Autodesk Inventor part; units mm, degrees
ref_plane "YZ Plane" through (0, 0, 0) normal (1, 0, 0) x (0, 1, 0)
ref_plane "XZ Plane" through (0, 0, 0) normal (0, 1, 0) x (-1, 0, 0)
ref_plane "XY Plane" through (0, 0, 0) normal (0, 0, 1) x (1, 0, 0)
sketch "Sketch1" plane through (0, 0, 0) normal (0, 0, 1) x (1, 0, 0)
  line L0 (-34.1, 30.847) -> (0, 30.847)
  line L1 (0, 33.247) -> (-34.1, 33.247)
  arc A0 (-0.8878, 31.7995) -> (0, 30.847) centre (0, 31.737) ccw
  line L2 (-3, 33.247) -> (-3, 30.847) construction
  line L3 (-7.3, 30.847) -> (-2.1, 30.847)
  line L4 (0, 30.847) -> (-34.1, 30.847) construction
  line L5 (0, 33.247) -> (0, 30.847)
  arc A1 (-3, 30.847) -> (-2.1122, 31.7995) centre (-3, 31.737) ccw
  line L6 (-34.1, 32.067) -> (-3, 32.067) construction
  line L7 (-1.8628, 32.067) -> (-1.1372, 32.067)
  arc A2 (-1.8628, 32.067) -> (-2.1122, 31.7995) centre (-1.8628, 31.817) ccw
  arc A3 (-0.8878, 31.7995) -> (-1.1372, 32.067) centre (-1.1372, 31.817) ccw
  arc A4 (-3.8878, 31.7995) -> (-3, 30.847) centre (-3, 31.737) ccw
  arc A5 (-3.8878, 31.7995) -> (-4.1372, 32.067) centre (-4.1372, 31.817) ccw
  line L8 (-4.1372, 32.067) -> (-4.8628, 32.067)
  arc A6 (-4.8628, 32.067) -> (-5.1122, 31.7995) centre (-4.8628, 31.817) ccw
  arc A7 (-6, 30.847) -> (-5.1122, 31.7995) centre (-6, 31.737) ccw
  line L9 (-6, 33.247) -> (-6, 30.847) construction
  line L10 (-9, 33.247) -> (-9, 30.847) construction
  arc A8 (-9, 30.847) -> (-8.1122, 31.7995) centre (-9, 31.737) ccw
  arc A9 (-7.8628, 32.067) -> (-8.1122, 31.7995) centre (-7.8628, 31.817) ccw
  line L11 (-7.1372, 32.067) -> (-7.8628, 32.067)
  arc A10 (-6.8878, 31.7995) -> (-7.1372, 32.067) centre (-7.1372, 31.817) ccw
  arc A11 (-6.8878, 31.7995) -> (-6, 30.847) centre (-6, 31.737) ccw
  line L12 (-12, 33.247) -> (-12, 30.847) construction
  arc A12 (-12, 30.847) -> (-11.1122, 31.7995) centre (-12, 31.737) ccw
  arc A13 (-10.8628, 32.067) -> (-11.1122, 31.7995) centre (-10.8628, 31.817) ccw
  line L13 (-10.1372, 32.067) -> (-10.8628, 32.067)
  arc A14 (-9.8878, 31.7995) -> (-10.1372, 32.067) centre (-10.1372, 31.817) ccw
  arc A15 (-9.8878, 31.7995) -> (-9, 30.847) centre (-9, 31.737) ccw
  line L14 (-15, 33.247) -> (-15, 30.847) construction
  arc A16 (-15, 30.847) -> (-14.1122, 31.7995) centre (-15, 31.737) ccw
  arc A17 (-13.8628, 32.067) -> (-14.1122, 31.7995) centre (-13.8628, 31.817) ccw
  line L15 (-13.1372, 32.067) -> (-13.8628, 32.067)
  arc A18 (-12.8878, 31.7995) -> (-13.1372, 32.067) centre (-13.1372, 31.817) ccw
  arc A19 (-12.8878, 31.7995) -> (-12, 30.847) centre (-12, 31.737) ccw
  line L16 (-18, 33.247) -> (-18, 30.847) construction
  arc A20 (-18, 30.847) -> (-17.1122, 31.7995) centre (-18, 31.737) ccw
  arc A21 (-16.8628, 32.067) -> (-17.1122, 31.7995) centre (-16.8628, 31.817) ccw
  line L17 (-16.1372, 32.067) -> (-16.8628, 32.067)
  arc A22 (-15.8878, 31.7995) -> (-16.1372, 32.067) centre (-16.1372, 31.817) ccw
  arc A23 (-15.8878, 31.7995) -> (-15, 30.847) centre (-15, 31.737) ccw
  line L18 (-21, 33.247) -> (-21, 30.847) construction
  arc A24 (-21, 30.847) -> (-20.1122, 31.7995) centre (-21, 31.737) ccw
  arc A25 (-19.8628, 32.067) -> (-20.1122, 31.7995) centre (-19.8628, 31.817) ccw
  line L19 (-19.1372, 32.067) -> (-19.8628, 32.067)
  arc A26 (-18.8878, 31.7995) -> (-19.1372, 32.067) centre (-19.1372, 31.817) ccw
  arc A27 (-18.8878, 31.7995) -> (-18, 30.847) centre (-18, 31.737) ccw
  line L20 (-24, 33.247) -> (-24, 30.847) construction
  arc A28 (-24, 30.847) -> (-23.1122, 31.7995) centre (-24, 31.737) ccw
  arc A29 (-22.8628, 32.067) -> (-23.1122, 31.7995) centre (-22.8628, 31.817) ccw
  line L21 (-22.1372, 32.067) -> (-22.8628, 32.067)
  arc A30 (-21.8878, 31.7995) -> (-22.1372, 32.067) centre (-22.1372, 31.817) ccw
  arc A31 (-21.8878, 31.7995) -> (-21, 30.847) centre (-21, 31.737) ccw
  line L22 (-27, 33.247) -> (-27, 30.847) construction
  arc A32 (-27, 30.847) -> (-26.1122, 31.7995) centre (-27, 31.737) ccw
  arc A33 (-25.8628, 32.067) -> (-26.1122, 31.7995) centre (-25.8628, 31.817) ccw
  line L23 (-25.1372, 32.067) -> (-25.8628, 32.067)
  arc A34 (-24.8878, 31.7995) -> (-25.1372, 32.067) centre (-25.1372, 31.817) ccw
  arc A35 (-24.8878, 31.7995) -> (-24, 30.847) centre (-24, 31.737) ccw
  line L24 (-30, 33.247) -> (-30, 30.847) construction
  arc A36 (-30, 30.847) -> (-29.1122, 31.7995) centre (-30, 31.737) ccw
  arc A37 (-28.8628, 32.067) -> (-29.1122, 31.7995) centre (-28.8628, 31.817) ccw
  line L25 (-28.1372, 32.067) -> (-28.8628, 32.067)
  arc A38 (-27.8878, 31.7995) -> (-28.1372, 32.067) centre (-28.1372, 31.817) ccw
  arc A39 (-27.8878, 31.7995) -> (-27, 30.847) centre (-27, 31.737) ccw
  line L26 (-33, 33.247) -> (-33, 30.847) construction
  arc A40 (-33, 30.847) -> (-32.1122, 31.7995) centre (-33, 31.737) ccw
  arc A41 (-31.8628, 32.067) -> (-32.1122, 31.7995) centre (-31.8628, 31.817) ccw
  line L27 (-31.1372, 32.067) -> (-31.8628, 32.067)
  arc A42 (-30.8878, 31.7995) -> (-31.1372, 32.067) centre (-31.1372, 31.817) ccw
  arc A43 (-30.8878, 31.7995) -> (-30, 30.847) centre (-30, 31.737) ccw
  line L28 (-36, 33.247) -> (-36, 30.847) construction
  arc A44 (-36, 30.847) -> (-35.1122, 31.7995) centre (-36, 31.737) ccw
  arc A45 (-34.8628, 32.067) -> (-35.1122, 31.7995) centre (-34.8628, 31.817) ccw
  line L29 (-34.1372, 32.067) -> (-34.8628, 32.067)
  arc A46 (-33.8878, 31.7995) -> (-34.1372, 32.067) centre (-34.1372, 31.817) ccw
  arc A47 (-33.8878, 31.7995) -> (-33, 30.847) centre (-33, 31.737) ccw
  line L30 (-34.1, 30.847) -> (-34.1, 33.247)
  line L31 (-34.1, 30.847) -> (0, 30.847)
  line L32 (0, 30.847) -> (0, 27.847)
  line L33 (0, 27.847) -> (-34.1, 27.847)
  line L34 (-34.1, 27.847) -> (-34.1, 30.847)
  point P0 (0, 0)
  point P1 (0, 20)
  point P2 (-0.8266, 32.067)
  point P3 (-2.1734, 32.067)
  point P4 (-34.1, 32.0642)
  point P5 (-34.1, 32.0642)
  dimension "d4" = 2.4
  dimension "d5" = 1.78
  dimension "d6" = 3
  dimension "d7" = 1.78
  dimension "d8" = 0.25
  dimension "d9" = 0.25
  dimension "d10" = 3
  dimension "d12" = 3
extrude "Extrusion1" add sketch "Sketch1" against normal blind 16 contours L30 A46 A47 L0 | L0 L32 L33 L34 | A40 A41 L27 A42 A43 L0 | A36 A37 L25 A38 A39 L0 | A32 A33 L23 A34 A35 L0 | L0 A1 A2 L7 A3 A0 | A28 A29 L21 A30 A31 L0 | A24 A25 L19 A26 A27 L0 | L0 A7 A6 L8 A5 A4 | A20 A21 L17 A22 A23 L0 | L0 A8 A9 L11 A10 A11 | A16 A17 L15 A18 A19 L0 | A12 A13 L13 A14 A15 L0
sketch "Sketch2" plane through (0, 27.847, 0) normal (1, 0, 0) x (0, 0, -1)
  line L0 (0, 0) -> (0, 3)
  line L1 (0, 0) -> (16, 0)
  line L2 (16, 3) -> (16, 0)
  line L3 (0, 3) -> (16, 3)
  line L4 (0, 0) -> (16, 0) construction
  line L5 (8, 0) -> (8, -9.1602) construction
  circle A0 centre (8, -1.5) radius 4.8
  circle A1 centre (8, -1.5) radius 2.6
  point P0 (0, -27.847)
  point P1 (5.8763, 0)
  point P2 (3.4404, 0)
  point P3 (12.5596, 0)
  point P4 (10.1237, 0)
  dimension "d15" = 9.6
  dimension "d16" = 1.5
  dimension "d17" = 5.2
extrude "Extrusion2" add sketch "Sketch2" against normal up to surface (34.1 mm away) contours L1 A1 A0
sketch "Sketch3" plane through (0, 27.847, 0) normal (1, 0, 0) x (0, 0, -1)
  arc A0 (5.8763, 0) -> (10.1237, 0) centre (8, -1.5) ccw
  line L0 (5.8763, 0) -> (10.1237, 0)
  circle A1 centre (8, -1.5) radius 2.6
  point P0 (0, -27.847)
extrude "Extrusion3" cut sketch "Sketch3" against normal through all contours A1 L0
sketch "Sketch4" plane through (-34.1, 27.847, -16) normal (0, -1, 0) x (1, 0, 0)
  line L0 (33.21, 16) -> (34.1, 16)
  line L1 (34.1, 16) -> (0, 16)
  line L2 (0, 16) -> (0, 28)
  line L3 (0, 28) -> (34.1, 28)
  line L4 (34.1, 28) -> (34.1, 16)
  line L5 (34.1, 3.4404) -> (34.1, 0)
  line L6 (34.1, 0) -> (0, 0)
  line L7 (0, 0) -> (0, -12)
  line L8 (0, -12) -> (34.1, -12)
  line L9 (34.1, -12) -> (34.1, 0)
  line L10 (34.1, 22) -> (0, 22) construction
  line L11 (34.1, -6) -> (0, -6) construction
  line L12 (27.05, 22) -> (7.05, 22) construction
  line L13 (7.05, 22) -> (7.05, -6) construction
  line L14 (7.05, -6) -> (27.05, -6) construction
  line L15 (27.05, -6) -> (27.05, 22) construction
  line L16 (23, 24.3383) -> (27.05, 26.6765)
  line L17 (27.05, 26.6765) -> (31.1, 24.3383)
  line L18 (31.1, 24.3383) -> (31.1, 19.6617)
  line L19 (31.1, 19.6617) -> (27.05, 17.3235)
  line L20 (27.05, 17.3235) -> (23, 19.6617)
  line L21 (23, 19.6617) -> (23, 24.3383)
  line L22 (31.1, -3.6617) -> (31.1, -8.3383)
  line L23 (27.05, -1.3235) -> (31.1, -3.6617)
  line L24 (23, -3.6617) -> (27.05, -1.3235)
  line L25 (23, -8.3383) -> (23, -3.6617)
  line L26 (27.05, -10.6765) -> (23, -8.3383)
  line L27 (31.1, -8.3383) -> (27.05, -10.6765)
  line L28 (11.1, 24.3383) -> (11.1, 19.6617)
  line L29 (7.05, 26.6765) -> (11.1, 24.3383)
  line L30 (3, 24.3383) -> (7.05, 26.6765)
  line L31 (3, 19.6617) -> (3, 24.3383)
  line L32 (7.05, 17.3235) -> (3, 19.6617)
  line L33 (11.1, 19.6617) -> (7.05, 17.3235)
  line L34 (11.1, -3.6617) -> (11.1, -8.3383)
  line L35 (7.05, -1.3235) -> (11.1, -3.6617)
  line L36 (3, -3.6617) -> (7.05, -1.3235)
  line L37 (3, -8.3383) -> (3, -3.6617)
  line L38 (7.05, -10.6765) -> (3, -8.3383)
  line L39 (11.1, -8.3383) -> (7.05, -10.6765)
  point P0 (33.2122, 16)
  point P1 (23, 22)
  point P2 (23, -6)
  point P3 (3, 22)
  point P4 (3, -6)
  dimension "d22" = 12
  dimension "d23" = 12
  dimension "d24" = 4.05
  dimension "d25" = 20
  dimension "d26" = 7.05
  dimension "d29" = 28
  dimension "d32" = 20
extrude "Extrusion4" add sketch "Sketch4" against normal blind 3
sketch "Sketch5" plane through (-34.1, 30.847, -16) normal (0, 1, 0) x (1, 0, 0)
  line L0 (3, -19.6617) -> (3, -24.3383) construction
  line L1 (3, -22) -> (11.1, -22) construction
  line L2 (11.1, -24.3383) -> (11.1, -19.6617) construction
  line L3 (23, 3.6617) -> (23, 8.3383) construction
  line L4 (23, 6) -> (31.1, 6) construction
  line L5 (31.1, 8.3383) -> (31.1, 3.6617) construction
  line L6 (7.05, -22) -> (27.05, -22) construction
  line L7 (27.05, -22) -> (27.05, 6) construction
  line L8 (27.05, 6) -> (7.05, 6) construction
  line L9 (7.05, 6) -> (7.05, -22) construction
  circle A0 centre (7.05, -22) radius 2.6
  circle A1 centre (7.05, 6) radius 2.6
  circle A2 centre (27.05, -22) radius 2.6
  circle A3 centre (27.05, 6) radius 2.6
  line L10 (0, -16) -> (0, -28)
  line L11 (0, -16) -> (0, 0)
  line L12 (0, 12) -> (0, 0)
  line L13 (34.1, 12) -> (0, 12)
  line L14 (34.1, 0) -> (34.1, 12)
  line L15 (34.1, -16) -> (34.1, 0)
  line L16 (34.1, -28) -> (34.1, -16)
  line L17 (0, -28) -> (34.1, -28)
  line L18 (0, -28) -> (34.1, -28)
  line L19 (34.1, -28) -> (34.1, -16)
  line L20 (31.1, -16) -> (34.1, -16)
  line L21 (28.1, -16) -> (31.1, -16)
  line L22 (25.1, -16) -> (28.1, -16)
  line L23 (22.1, -16) -> (25.1, -16)
  line L24 (19.1, -16) -> (22.1, -16)
  line L25 (16.1, -16) -> (19.1, -16)
  line L26 (13.1, -16) -> (16.1, -16)
  line L27 (10.1, -16) -> (13.1, -16)
  line L28 (7.1, -16) -> (10.1, -16)
  line L29 (4.1, -16) -> (7.1, -16)
  line L30 (1.1, -16) -> (4.1, -16)
  line L31 (0, -16) -> (1.1, -16)
  line L32 (0, -16) -> (0, -28)
  line L33 (11.1, -19.6617) -> (11.1, -24.3383)
  line L34 (11.1, -24.3383) -> (7.05, -26.6765)
  line L35 (7.05, -26.6765) -> (3, -24.3383)
  line L36 (3, -24.3383) -> (3, -19.6617)
  line L37 (3, -19.6617) -> (7.05, -17.3235)
  line L38 (7.05, -17.3235) -> (11.1, -19.6617)
  line L39 (27.05, -26.6765) -> (23, -24.3383)
  line L40 (23, -24.3383) -> (23, -19.6617)
  line L41 (23, -19.6617) -> (27.05, -17.3235)
  line L42 (27.05, -17.3235) -> (31.1, -19.6617)
  line L43 (31.1, -19.6617) -> (31.1, -24.3383)
  line L44 (31.1, -24.3383) -> (27.05, -26.6765)
  line L45 (34.1, 12) -> (0, 12)
  line L46 (0, 12) -> (0, 0)
  line L47 (1.1, 0) -> (0, 0)
  line L48 (4.1, 0) -> (1.1, 0)
  line L49 (7.1, 0) -> (4.1, 0)
  line L50 (10.1, 0) -> (7.1, 0)
  line L51 (13.1, 0) -> (10.1, 0)
  line L52 (16.1, 0) -> (13.1, 0)
  line L53 (19.1, 0) -> (16.1, 0)
  line L54 (22.1, 0) -> (19.1, 0)
  line L55 (25.1, 0) -> (22.1, 0)
  line L56 (28.1, 0) -> (25.1, 0)
  line L57 (31.1, 0) -> (28.1, 0)
  line L58 (34.1, 0) -> (31.1, 0)
  line L59 (34.1, 0) -> (34.1, 12)
  line L60 (11.1, 8.3383) -> (11.1, 3.6617)
  line L61 (11.1, 3.6617) -> (7.05, 1.3235)
  line L62 (7.05, 1.3235) -> (3, 3.6617)
  line L63 (3, 3.6617) -> (3, 8.3383)
  line L64 (3, 8.3383) -> (7.05, 10.6765)
  line L65 (7.05, 10.6765) -> (11.1, 8.3383)
  line L66 (31.1, 8.3383) -> (31.1, 3.6617)
  line L67 (31.1, 3.6617) -> (27.05, 1.3235)
  line L68 (27.05, 1.3235) -> (23, 3.6617)
  line L69 (23, 3.6617) -> (23, 8.3383)
  line L70 (23, 8.3383) -> (27.05, 10.6765)
  line L71 (27.05, 10.6765) -> (31.1, 8.3383)
  dimension "d37" = 5.2
  dimension "d38" = 5.2
  dimension "d39" = 5.2
  dimension "d40" = 5.2
extrude "Extrusion5" add sketch "Sketch5" along normal up to surface (1.22 mm away) contours L31 L30 L29 L28 L27 L26 L25 L24 L23 L22 L21 L20 L16 L17 L10 | L12 L13 L14 L58 L57 L56 L55 L54 L53 L52 L51 L50 L49 L48 L47 | L33 L34 L35 L36 L37 L38 | L39 L40 L41 L42 L43 L44 | L60 L61 L62 L63 L64 L65 | L66 L67 L68 L69 L70 L71
equation "\"d7\" = d5"
equation "\"d23\" = d22"
properties part number "Y Axis Belt Adjustable Grip Plate"
Part model, mm, in its own coordinate system. A direction names the side the tool comes from. Give positions to 0.01 mm unless a question says otherwise; leave off trailing zeros. Order: outer loops, then holes, each group sorted by start corner. A loop starts at its lowest first (then second) coordinate and runs counter-clockwise, first axis right, second up. Notation, with made-up numbers: (76, 72.25) - (131, 72.25) arc R24 ccw to (131, 85.25) - close; hole circle Ø1 at (38, 72). An arc over 180 degrees is marked (long way). One line per question, with ' | ' between items.
1. Band-saw the part on B-B on y = 27. List the corners of the cut face in (x, z).
Filled in:
outline: (-34.1, -12.76) - (0, -12.76) - (0, -10.52) - (-34.1, -10.52) - close; (-34.1, -5.48) - (0, -5.48) - (0, -3.24) - (-34.1, -3.24) - close
2. Band-saw the part on C-C on z = 6.5. List the corners of the cut face in (x, y), then the cut area to 3 significant figures.
Filled in:
outline: (-34.1, 27.85) - (-31.1, 27.85) - (-31.1, 30.85) - (-29.6, 30.85) - (-29.6, 32.07) - (-34.1, 32.07) - close; (-24.5, 30.85) - (-23, 30.85) - (-23, 27.85) - (-11.1, 27.85) - (-11.1, 30.85) - (-9.6, 30.85) - (-9.6, 32.07) - (-24.5, 32.07) - close; (-4.5, 30.85) - (-3, 30.85) - (-3, 27.85) - (0, 27.85) - (0, 32.07) - (-4.5, 32.07) - close | area: 82.9 mm²
3. Which spindle directions (+Z, -Z, +X, -X, +Y, -Y) get a long thin tool onto all of the face, cutting with end or side? Do faces 3 (the face through (-0.4, 31.6, -16)), 4 (the face through (-7.388, 31.448, -19.422)), 5 (the face through (-25.05, 29.33, 9.52)), 6 (the face through (-33, 31, -16)). Say none if no direction does.
Filled in:
face 3: +X, +Y | face 4: +Y, -Y | face 5: -Y | face 6: +Y
4. Drill centre lines: probe 1 along X at (y, z) = (31.5, 6); probe 2 along Z at (x, y) = (-27.05, 31.15); probe 3 along Z at (x, y) = (-7.05, 31.15). Where is each one in solid material? Low to high.
Filled in:
probe 1: -34.1 to -29.65, -24.45 to -9.65, -4.45 to 0 | probe 2: -28 to -24.6, -19.4 to -16, 0 to 3.4, 8.6 to 12 | probe 3: -28 to -24.6, -19.4 to 3.4, 8.6 to 12
5. Drop flat-ended pins along their axis: P1, Ø6.5, axis at x = -8, z = -19.5, coming from the -Y side; P2, Ø4, axis at y = 26.347, z = -8, coming from the -X side; P3, Ø1.5, axis at x = -27.5, y = 24, coming from the -Z side; P4, Ø2.5, axis at y = 29.5, z = -23, coming from the +X side. Give the stop position or say it passes through.
Filled in:
P1: y = 27.85 | P2: through | P3: z = -12.53 | P4: x = 0
6. Pull direction Z, two halves, no side cores. Call faces 1 (the face through (-17, 30, -28)), 2 (the face through (-9, 31, -16)): +Z half, -Z half, draft (parallel to the pull), parting line (faces both ways), or undercut.
Filled in:
face 1: -Z half | face 2: undercut
7. Band-saw the part on A-A on z = -22. List the corners of the cut face in (x, y), then the cut area to 3 significant figures.
Filled in:
outline: (-34.1, 27.85) - (-31.1, 27.85) - (-31.1, 30.85) - (-29.65, 30.85) - (-29.65, 32.07) - (-34.1, 32.07) - close; (-24.45, 30.85) - (-23, 30.85) - (-23, 27.85) - (-11.1, 27.85) - (-11.1, 30.85) - (-9.65, 30.85) - (-9.65, 32.07) - (-24.45, 32.07) - close; (-4.45, 30.85) - (-3, 30.85) - (-3, 27.85) - (0, 27.85) - (0, 32.07) - (-4.45, 32.07) - close | area: 82.6 mm²
